The drawing under review shows one solid part. Ordinate dimensions are in mm from its lowest x, y, z. Coordinates: 2 decimals unless noted, no trailing zeros. Loops run counter-clockwise (first coordinate to the right, second up) from the corner with the lowest first, then second, coordinate; pieces in that order, holes last. Notation, with made-up numbers: M -13.5,86 L 5.5,86 A13 cw 5.5,101 Z; hole C -30.5,13.5 d10. An arc over 180 degrees is marked long. Use one line per item in the form item = value.
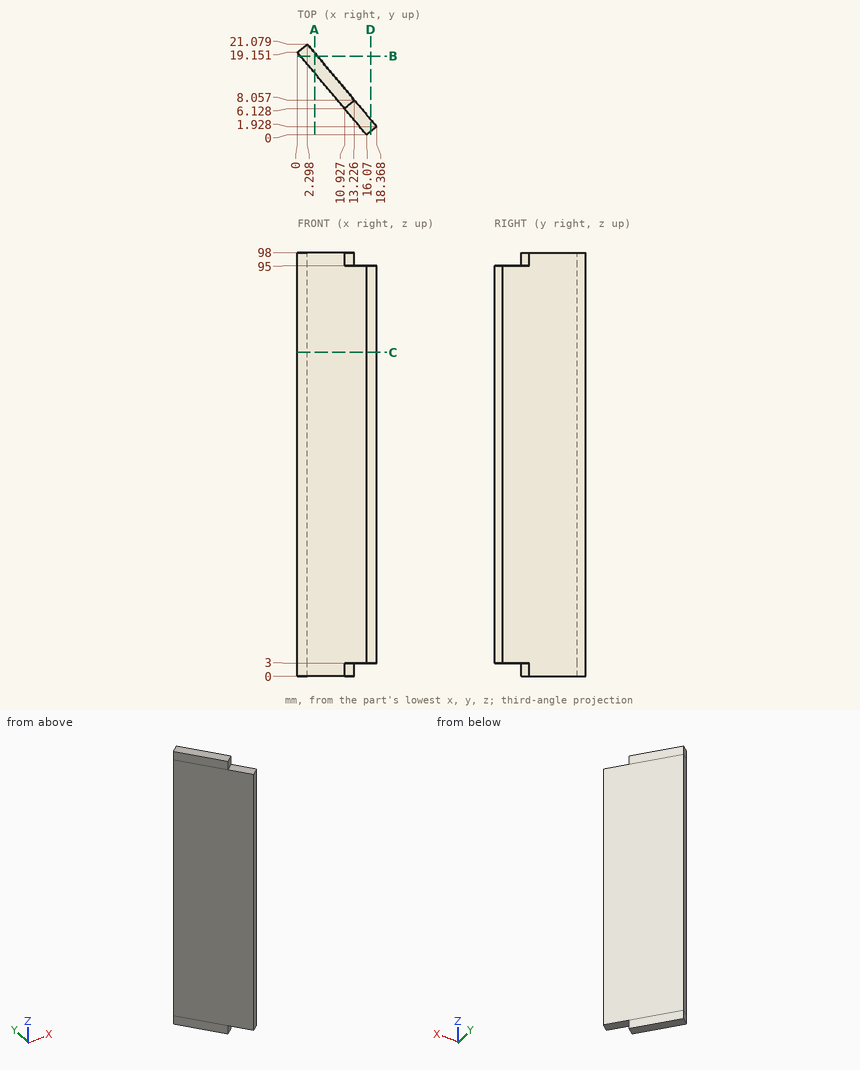
1. For pin 1 Ø8 at (y, z) = (12, 79.5) entering from +X; pin 2 Ø6 at (x, y) = (14, 4.5) entering from -Z; pin 3 Ø3.5 at (x, y) = (13.5, 4) entering from +Z; pin 4 Ø2 at (x, y) = (8, 17) entering from -Z, all flat-tipped, find the tip position at first contact; note any pin that passes through.
Computed values:
pin_1 = 13.27
pin_2 = 3
pin_3 = 95
pin_4 = through
2. Consider section B-B on y = 18.25. Write out the cut boundary in (x, z), plus the area to 3 significant figures.
Computed values:
outline = M 0.76,0 L 4.67,0 L 4.67,98 L 0.76,98 Z
area = 384 mm2
3. Wall thickness on line 1 along X through (y, z) = (14.5, 74.5) (1 decimal); line 2 along Y through (x, z) = (2, 15) (1 decimal); line 3 along X through (y, z) = (15.5, 87.5) (1 decimal): over which ranges is each line inside the solid? List them lowest first. Write a range as from..to.
Computed values:
line_1 = 3.9..7.8
line_2 = 16.8..20.8
line_3 = 3.1..7
4. Consider section A-A on x = 4. Write out the cut boundary in (y, z) (1 decimal).
Computed values:
outline = M 14.4,0 L 19.1,0 L 19.1,98 L 14.4,98 Z
5. Consider section C-C on z = 75. Write out the cut boundary in (x, y).
Computed values:
outline = M 0,19.15 L 16.07,0 L 18.37,1.93 L 2.3,21.08 Z
6. Consider section D-D on x = 17. Write out the cut boundary in (y, z).
Computed values:
outline = M 0.78,3 L 3.56,3 L 3.56,95 L 0.78,95 Z
